```python
from build123d import *

# Parameters (mm, degrees)
SKETCH070_W     = 11.35
SKETCH070_H     = 17.44
PAD008_DEPTH    = 1
SKETCH071_W     = 5
SKETCH071_H     = 5
SKETCH071_H_2   = 4.5
PAD009_DEPTH    = 1
SKETCH077_W     = 6.5
SKETCH077_H     = 1.5
POCKET030_DEPTH = 5
SKETCH090_W     = 22
SKETCH090_H     = 28
PAD021_DEPTH    = 1
FILLET016_R     = 0.4


with BuildPart() as part:
    # Sketch070 → Pad008 (new body)
    with BuildSketch(Plane.XY):
        with BuildLine():
            Line((-9.548198, 6.6), (9.548198, 6.6))
            Line((9.548198, 6.6), (24.582245, -30.129227))
            ThreePointArc((24.582245, -30.129227), (21.935707, -33.270294), (22.144365, -37.372358))
            Line((29.035486, -54.207849), (22.144365, -37.372358))
            Line((25.057074, -60.930809), (29.035486, -54.207849))
            Line((29.76445, -70.068592), (25.057074, -60.930809))
            Line((23.9869, -75.767923), (29.76445, -70.068592))
            Line((12.771037, -90.465016), (23.9869, -75.767923))
            Line((10.366563, -90.465016), (12.771037, -90.465016))
            ThreePointArc((10.366563, -90.465016), (8.6, -87.040094), (5, -85.665016))
            Line((-5, -85.665016), (5, -85.665016))
            ThreePointArc((-5, -85.665016), (-8.6, -87.040094), (-10.366563, -90.465016))
            Line((-12.771037, -90.465016), (-10.366563, -90.465016))
            Line((-23.9869, -75.767923), (-12.771037, -90.465016))
            Line((-29.76445, -70.068592), (-23.9869, -75.767923))
            Line((-25.057074, -60.930809), (-29.76445, -70.068592))
            Line((-29.035486, -54.207849), (-25.057074, -60.930809))
            Line((-22.144365, -37.372358), (-29.035486, -54.207849))
            ThreePointArc((-22.144365, -37.372358), (-21.935707, -33.270294), (-24.582245, -30.129227))
            Line((-24.582245, -30.129227), (-9.548198, 6.6))
        make_face()
        with Locations((0.005, -59.43)):
            Rectangle(SKETCH070_W, SKETCH070_H, mode=Mode.SUBTRACT)
    extrude(amount=PAD008_DEPTH)

    # Sketch071 (on Face26 of Pad008) → Pad009 (join)
    with BuildSketch(Plane.XY.offset(1)):
        with Locations((-5.913956, 6.9)):
            Rectangle(SKETCH071_W, SKETCH071_H)
        with Locations((5.913956, 6.9)):
            Rectangle(SKETCH071_W, SKETCH071_H)
        with Locations((0, -85.915016)):
            Rectangle(SKETCH071_W, SKETCH071_H_2)
    extrude(amount=PAD009_DEPTH)

    # Sketch077 (on Face5 of Pad009) → Pocket030 (cut)
    with BuildSketch(Plane.XY.offset(1)):
        with Locations((-0.45, -81.465016)):
            Rectangle(SKETCH077_W, SKETCH077_H)
    extrude(amount=-POCKET030_DEPTH, mode=Mode.SUBTRACT)

    # Sketch090 (on Face5 of Pocket030) → Pad021 (join)
    with BuildSketch(Plane.XY.offset(1)):
        with BuildLine():
            Line((-9.413956, 6.4), (9.413956, 6.4))
            Line((9.413956, 6.4), (24.582245, -30.129227))
            ThreePointArc((24.582245, -30.129227), (21.935707, -33.270294), (22.144365, -37.372358))
            Line((22.144365, -37.372358), (29.035486, -54.207849))
            Line((29.035486, -54.207849), (25.057074, -60.930809))
            Line((25.057074, -60.930809), (29.76445, -70.068592))
            Line((29.76445, -70.068592), (23.9869, -75.767923))
            Line((23.9869, -75.767923), (12.771037, -90.465016))
            Line((12.771037, -90.465016), (10.366563, -90.465016))
            ThreePointArc((10.366563, -90.465016), (8.6, -87.040094), (5, -85.665016))
            Line((-5, -85.665016), (5, -85.665016))
            ThreePointArc((-5, -85.665016), (-8.6, -87.040094), (-10.366563, -90.465016))
            Line((-10.366563, -90.465016), (-12.771037, -90.465016))
            Line((-12.771037, -90.465016), (-23.9869, -75.767923))
            Line((-23.9869, -75.767923), (-29.76445, -70.068592))
            Line((-29.76445, -70.068592), (-25.057074, -60.930809))
            Line((-25.057074, -60.930809), (-29.035486, -54.207849))
            Line((-29.035486, -54.207849), (-22.144365, -37.372358))
            ThreePointArc((-22.144365, -37.372358), (-21.935707, -33.270294), (-24.582245, -30.129227))
            Line((-24.582245, -30.129227), (-9.413956, 6.4))
        make_face()
        with BuildLine():
            Line((-8.746409, 5.4), (8.746409, 5.4))
            Line((8.746409, 5.4), (23.336592, -29.736995))
            ThreePointArc((23.336592, -29.736995), (20.922218, -33.157742), (21.051699, -37.342708))
            Line((21.985036, -39.622914), (21.051699, -37.342708))
            Line((12, -43.71), (21.985036, -39.622914))
            Line((-12, -43.71), (12, -43.71))
            Line((-21.985036, -39.622914), (-12, -43.71))
            Line((-21.225759, -37.767948), (-21.985036, -39.622914))
            ThreePointArc((-21.225759, -37.767948), (-20.859949, -33.37892), (-23.336592, -29.736995))
            Line((-8.746409, 5.4), (-23.336592, -29.736995))
        make_face(mode=Mode.SUBTRACT)
        Polygon((-27.921656, -54.126491), (-23.914923, -60.897309), (-28.538789, -69.872986), (-23.234585, -75.10538), (-20.25505, -79.009716), (-12, -72.71), (-12, -44.790529), (-22.363851, -40.548387), align=None, mode=Mode.SUBTRACT)
        with BuildLine():
            Line((12.276247, -89.465016), (19.648388, -79.804676))
            Line((19.648388, -79.804676), (11.662019, -73.71))
            Line((11.662019, -73.71), (-11.662019, -73.71))
            Line((-11.662019, -73.71), (-19.648388, -79.804676))
            Line((-19.648388, -79.804676), (-12.276247, -89.465016))
            Line((-12.276247, -89.465016), (-11.196773, -89.465016))
            ThreePointArc((-5, -84.665016), (-8.919184, -86.005372), (-11.196773, -89.465016))
            Line((-5, -84.665016), (5, -84.665016))
            ThreePointArc((11.196773, -89.465016), (8.919184, -86.005372), (5, -84.665016))
            Line((11.196773, -89.465016), (12.276247, -89.465016))
        make_face(mode=Mode.SUBTRACT)
        Polygon((23.234585, -75.10538), (28.538789, -69.872986), (23.914923, -60.897309), (27.921656, -54.126491), (22.363851, -40.548387), (12, -44.790529), (12, -72.71), (20.25505, -79.009716), align=None, mode=Mode.SUBTRACT)
        with Locations((0, -58.71)):
            Rectangle(SKETCH090_W, SKETCH090_H, mode=Mode.SUBTRACT)
    extrude(amount=PAD021_DEPTH)

    # Fillet016
    fillet016_edges = [part.edges().sort_by_distance(p)[0] for p in [
        (0, -88.165016, 2),
        (0, -88.165016, 1),
        (0, -83.665016, 2),
        (-5.913956, 4.4, 2),
        (5.913956, 4.4, 2),
        (5.913956, 9.4, 2),
        (-5.913956, 9.4, 2),
        (-5.913956, 9.4, 1),
        (5.913956, 9.4, 1),
        (-11.5688, -90.465016, 2),
        (11.5688, -90.465016, 2),
        (0, 6.4, 2),
    ]]
    fillet(fillet016_edges, radius=FILLET016_R)


with BuildPart() as part_1:
    # Body005 placement: moved
    add(part.part.moved(Location((0, 0, 0.5))))


solid = part_1.part
```
CAD build for the part. Positions are in the model's coordinates, mm. A direction names the side the tool comes from. Round coordinates to 2 decimals unless told otherwise and drop trailing zeros. Write each loop counter-clockwise with the first axis right and the second up, starting at its lowest first coordinate (ties: lowest second). Pieces come first, ordered by that corner, then holes. Notation, with made-up numbers: (75, 33.5) - (133, 33.5) arc R30 ccw to (133, 67.5) - close; hole circle Ø3 at (84, 25.25). An arc over 180 degrees is marked (long way). Write item = value, one per line. Start each with the question number.
Q1. Probe L1, parallel to Y at x = 1, z = 2.15; L2, parallel to Y at x = -2.5, z = 0.95; L3, parallel to X at y = -74, z = 1.8. List the from-to ranges inside material, lowest first. Write a range as from..to.
Q2. Mould opens along X. For faces 6 (the cylindrical face through (-8.559, -87.004, 1.486)), 7 (the flat face through (6, 8, 1.5)), 8 (the flat face through (-17.104, -12.12, 1.993)) say: pulls with the +X half, pulls with the -X half, needs draft (parallel to the pull), parting line crosses it, or undercut.
Q3. Drop flat-ended pins along their axis: pin 1 (0.5 mm diameter, centred on y = -57.5, z = 2, fed in from -X); pin 2 (0.5 mm diameter, centred on x = 2, z = 1, fed in from +Y); pin 3 (0.5 mm diameter, centred on y = -87, z = 2, fed in from -X). Give the stop position or say it passes through.
Q4. Which spindle directions (+Z, -Z, +X, -X, +Y, -Y) get a long thin tool onto all of the face, cutting with end or side? Do faces 1 (the flat face through (16.07, -75.816, 1.993)), 2 (the flat face through (16.892, -11.609, 1.993)), 3 (the cylindrical face through (8.641, -87.077, 1.486)), 4 (the flat face through (16.96, -11.51, 0.99)), 5 (the flat face through (-27.44, -65.56, 1.49)). Say none if no direction does.
Q5. Band-saw the part on B-B (x = 15). Give the cut face in (y, z).
Q6. Band-saw the part on A-A (y = -46.5). Give the cut face in (x, z), then the cut area to 3 significant figures.
Answers below:
q1.L1 = -88.16..-83.67, -73.71..-72.71, -44.71..-43.71, 5.4..6.4
q1.L2 = -85.67..-82.22, -80.72..-68.15, -50.71..6.6
q1.L3 = -25.78..-24.36, -13.69..-12.04, 12.04..13.69, 24.36..25.78
q2.face_6 = undercut
q2.face_7 = needs draft
q2.face_8 = pulls with the -X half
q3.pin_1 = -27.24
q3.pin_2 = 6.6
q3.pin_3 = -15.61
q4.face_1 = +Z
q4.face_2 = +Z, +X, +Y
q4.face_3 = +Z, -Z, -Y
q4.face_4 = +Z, -Z, +X, +Y
q4.face_5 = +Z, -Z, -X
q5.outline = (-87.54, 0.5) - (-6.72, 0.5) - (-6.72, 1.5) - (-7.05, 1.5) - (-7.05, 2.5) - (-9.66, 2.5) - (-9.66, 1.5) - (-42.48, 1.5) - (-42.48, 2.5) - (-43.56, 2.5) - (-43.56, 1.5) - (-75, 1.5) - (-75, 2.5) - (-76.26, 2.5) - (-76.26, 1.5) - (-85.9, 1.5) - (-85.9, 2.5) - (-87.54, 2.5) - close
q6.outline = (-25.88, 0.5) - (25.88, 0.5) - (25.88, 2.5) - (24.8, 2.5) - (24.8, 1.5) - (12, 1.5) - (12, 2.5) - (11, 2.5) - (11, 1.5) - (-11, 1.5) - (-11, 2.5) - (-12, 2.5) - (-12, 1.5) - (-24.8, 1.5) - (-24.8, 2.5) - (-25.88, 2.5) - close
q6.area = 55.9 mm2
